```python
from build123d import *

# Parameters (mm, degrees)
SKETCH1_W           = 35.4
SKETCH1_H           = 13.6
BOSS_EXTRUDE1_DEPTH = 1.825
SKETCH2_W           = 4.8
SKETCH2_H           = 12
BOSS_EXTRUDE2_DEPTH = 4.15
SKETCH3_W           = 4.8
SKETCH3_H           = 12
BOSS_EXTRUDE3_DEPTH = 4.15
SKETCH4_W           = 6
SKETCH4_H           = 1.25
REVOLVE1_ANGLE      = 180


with BuildPart() as part:
    # Sketch1 → Boss-Extrude1 (new, symmetric)
    with BuildSketch(Plane.XY):
        Rectangle(SKETCH1_W, SKETCH1_H)
    extrude(amount=BOSS_EXTRUDE1_DEPTH, both=True)

    # Sketch2 → Boss-Extrude2 (add)
    with BuildSketch(Plane.XY.offset(1.825)):
        with Locations((-15.3, 0)):
            Rectangle(SKETCH2_W, SKETCH2_H)
    extrude(amount=BOSS_EXTRUDE2_DEPTH)

    # Sketch3 → Boss-Extrude3 (add)
    with BuildSketch(Plane(origin=(0, 0, -1.825), x_dir=(-1, 0, 0), z_dir=(0, 0, -1))):
        with Locations((15.3, 0)):
            Rectangle(SKETCH3_W, SKETCH3_H)
    extrude(amount=BOSS_EXTRUDE3_DEPTH)

    # Sketch4 → Revolve1 (revolve)
    with BuildSketch(Plane(origin=(0, 0, -1.825), x_dir=(-1, 0, 0), z_dir=(0, 0, -1))):
        with Locations((-20.7, 0.625)):
            Rectangle(SKETCH4_W, SKETCH4_H)
        with Locations((-14.7, 0.625)):
            Rectangle(SKETCH4_W, SKETCH4_H)
    revolve(axis=Axis((11.7, 0, -1.825), (-1, 0, 0)), revolution_arc=REVOLVE1_ANGLE)


solid = part.part
```
Part model, mm, in its own coordinate system. A direction names the side the tool comes from. Give positions to 0.01 mm unless a question says otherwise; leave off trailing zeros. Order: outer loops, then holes, each group sorted by start corner. A loop starts at its lowest first (then second) coordinate and runs counter-clockwise, first axis right, second up. Notation, with made-up numbers: (41.5, 40.25) - (51.5, 40.25) arc R22 cw to (51.5, 63.25) - close; hole circle Ø7 at (57.5, -32.75). An arc over 180 degrees is marked (long way). Use one line per item in the form item = value.
Item 1: Slice it at D-D on y = 0. Give the cut face in (x, z) (3 decimals), and give its area (3 significant figures).
Solution:
outline = (-17.7, -5.975) - (-12.9, -5.975) - (-12.9, -1.825) - (11.7, -1.825) - (11.7, -3.075) - (23.7, -3.075) - (23.7, -1.825) - (17.7, -1.825) - (17.7, 1.825) - (-12.9, 1.825) - (-12.9, 5.975) - (-17.7, 5.975) - close
area = 184 mm2
Item 2: Slice it at C-C on z = 4. Give the cut face in (x, y), and give its area (3 significant figures).
Solution:
outline = (-17.7, -6) - (-12.9, -6) - (-12.9, 6) - (-17.7, 6) - close
area = 57.6 mm2
Item 3: Slice it at A-A on y = -4. Give the cut face in (x, z) (3 decimals), and give its area (3 significant figures).
Solution:
outline = (-17.7, -5.975) - (-12.9, -5.975) - (-12.9, -1.825) - (17.7, -1.825) - (17.7, 1.825) - (-12.9, 1.825) - (-12.9, 5.975) - (-17.7, 5.975) - close
area = 169 mm2
Item 4: Probe probe 1 along X at (y, z) = (1.25, -4); probe 2 along Z at (x, y) = (6, 2) (3 decimals); probe 3 along X at (y, z) = (5.25, 1.5). List the from-to ranges inside material, lowest first. Write a range as from..to.
Solution:
probe_1 = -17.7..-12.9
probe_2 = -1.825..1.825
probe_3 = -17.7..17.7
Item 5: Which spindle directions (+Z, -Z, +X, -X, +Y, -Y) get a long thin tool onto all of the face, cutting with end or side? Do faces 5 (the face through (-15, 6, -4)), 6 (the face through (21, 0, -1.825)), 7 (the face through (17.784, 0.027, -3.075)), 8 (the face through (-15, 6, 4)), 9 (the face through (-15, -6, -4)). Say none if no direction does.
Solution:
face_5 = -Z, +X, -X, +Y
face_6 = +Z, +X, +Y, -Y
face_7 = -Z, +X
face_8 = +Z, +X, -X, +Y
face_9 = -Z, +X, -X, -Y
Item 6: Two-plate mould, pull along X, no slides. Class faces 1 (the face through (-15, -6, 4)), 2 (the face through (-17.7, 0, 0)), 3 (the face through (11.7, 0, -2)), 4 (the face through (17.7, 0, 0)): released by +X, released by -X, zero draft, split by the parting line, or undercut.
Solution:
face_1 = zero draft
face_2 = released by -X
face_3 = undercut
face_4 = released by +X
Item 7: Pin check, flat tips, straight feed: pin 1 Ø3 at (x, y) = (-9, 1) entering from -Z (3 decimals); pin 2 Ø2 at (y, z) = (1, -4) entering from +X; pin 3 Ø2 at (x, z) = (-1.5, -4) entering from +Y; pin 4 Ø4.5 at (x, z) = (-16, 4.5) entering from -Y. Stop position of each tip, or through.
Solution:
pin_1 = -1.825
pin_2 = -12.9
pin_3 = through
pin_4 = -6
Item 8: Slice it at B-B on x = -14. Give the cut face in (y, z) (3 decimals).
Solution:
outline = (-6.8, -1.825) - (-6, -1.825) - (-6, -5.975) - (6, -5.975) - (6, -1.825) - (6.8, -1.825) - (6.8, 1.825) - (6, 1.825) - (6, 5.975) - (-6, 5.975) - (-6, 1.825) - (-6.8, 1.825) - close
